The listing builds one solid part. Answer for the finished solid, in the listing's coordinates (mm). Face numbers are marked on the shaded views. A direction names the side the tool comes from. Give positions to 0.01 mm unless a question says otherwise; leave off trailing zeros. Write each loop counter-clockwise with the first axis right and the second up, starting at its lowest first coordinate (ties: lowest second). Pieces come first, ordered by that corner, then holes. Notation, with made-up numbers: (87, 72.5) - (116, 72.5) arc R12 ccw to (116, 76.5) - close; hole circle Ø4 at (-13.5, 57.25). An arc over 180 degrees is marked (long way). Return JSON: item names as keys, results as strings.
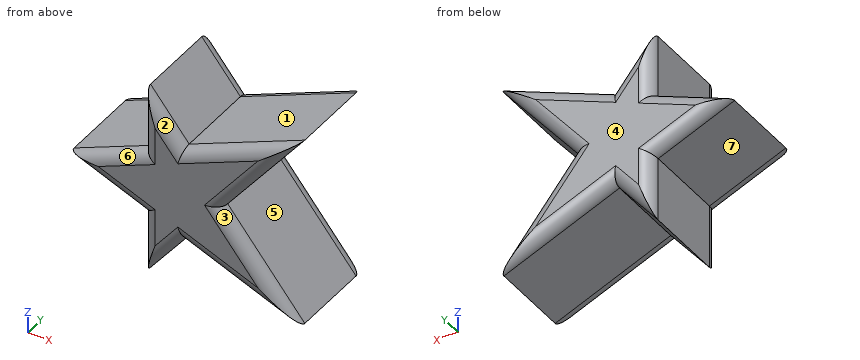
from build123d import *

# Parameters (mm, degrees)
F1_DEPTH = 22.225
F2_R     = 5.08


with BuildPart() as f1:
    # F0 (on Front) → F1 (new body, symmetric)
    with BuildSketch(Plane.XZ):
        Polygon((-0.2670160154, 19.9477417592), (-16.4844337851, 13.2459064213), (-16.4844337851, -13.2459064213), (-0.2670160154, -19.9477417592), (15.87390434, 0), align=None)
        Polygon((-16.4844337851, 13.2459064213), (-48.5375039279, 0), (-16.4844337851, -13.2459064213), align=None)
        Polygon((-16.4844337851, 39.9900227785), (-16.4844337851, 13.2459064213), (-0.2670160154, 19.9477417592), align=None)
        Polygon((48.232242465, 39.9900227785), (-0.2670160154, 19.9477417592), (15.87390434, 0), align=None)
        Polygon((15.87390434, 0), (-0.2670160154, -19.9477417592), (48.232242465, -39.9900227785), align=None)
        Polygon((-0.2670160154, -19.9477417592), (-16.4844337851, -13.2459064213), (-16.4844337851, -39.9900227785), align=None)
    extrude(amount=F1_DEPTH, both=True)

    # F2
    f2_edges = [f1.edges().sort_by_distance(p)[0] for p in [
        (-32.510969, -22.225, -6.622953),
        (-16.484434, -22.225, -26.617965),
        (-8.375725, -22.225, -29.968882),
        (23.982613, -22.225, -29.968882),
        (32.053073, -22.225, -19.995011),
        (32.053073, -22.225, 19.995011),
        (23.982613, -22.225, 29.968882),
        (-8.375725, -22.225, 29.968882),
        (-16.484434, -22.225, 26.617965),
        (-32.510969, -22.225, 6.622953),
        (-32.510969, 22.225, 6.622953),
        (-16.484434, 22.225, 26.617965),
        (-8.375725, 22.225, 29.968882),
        (23.982613, 22.225, 29.968882),
        (32.053073, 22.225, 19.995011),
        (32.053073, 22.225, -19.995011),
        (23.982613, 22.225, -29.968882),
        (-8.375725, 22.225, -29.968882),
        (-16.484434, 22.225, -26.617965),
        (-32.510969, 22.225, -6.622953),
    ]]
    fillet(f2_edges, radius=F2_R)


solid = f1.part
Item 1: Consider L1, parallel to X at y = -2, z = -21.5; L2, parallel to Z at x = 43, y = 2; L3, parallel to X at y = 18, z = -33. Determine where each line is inside the solid, lowest interval first.
Answer below:
{"L1": "x = -16.48 to -1.52, 3.49 to 33.27", "L2": "z = -37.83 to -33.52, 33.52 to 37.83", "L3": "x = -16.41 to -10.92, 31.51 to 42.48"}
Item 2: Flat-ended cylindrical pins translate along their axes: P1, Ø5, axis at y = -16, z = -9.5, coming from the +X side; P2, Ø4, axis at x = -10.5, y = 17, coming from the -Z side; P3, Ø8, axis at y = 14.5, z = -14, coming from the -X side. Find the tip coordinate at first contact, or state that the pin passes through.
Answer below:
{"P1": "stops at x = 25.58", "P2": "stops at z = -35.07", "P3": "stops at x = -24.34"}
Item 3: For the marked faces 1, 2 and 3, determine the directions among +Z, -Z, +X, -X, +Y, -Y from which every point of the face is accessible in a straight line to the end or side of a thin tool.
Answer below:
{"face 1": "+Z, +Y, -Y", "face 2": "+Z, -Y", "face 3": "+X, -Y"}
Item 4: A cutting plane is placed at B-B on y = 19. Determine the outline of the cut face in (x, z).
Answer below:
{"outline": "(-47.62, 0) - (-16.13, -13.01) - (-16.13, -39) - (-0.38, -19.52) - (47.09, -39.14) - (15.42, 0) - (47.09, 39.14) - (-0.38, 19.52) - (-16.13, 39) - (-16.13, 13.01) - close"}
Item 5: A cutting plane is placed at A-A on y = -9. Determine the outline of the cut face in (x, z).
Answer below:
{"outline": "(-48.54, 0) - (-16.48, -13.25) - (-16.48, -39.99) - (-0.27, -19.95) - (48.23, -39.99) - (15.87, 0) - (48.23, 39.99) - (-0.27, 19.95) - (-16.48, 39.99) - (-16.48, 13.25) - close"}
Item 6: The mould has two halves that part along Z. Classify the marked faces 4, 5, 6 and 7: +Z half, -Z half, draft (parallel to the pull), parting line (faces both ways), or undercut.
Answer below:
{"face 4": "draft", "face 5": "undercut", "face 6": "+Z half", "face 7": "-Z half"}
